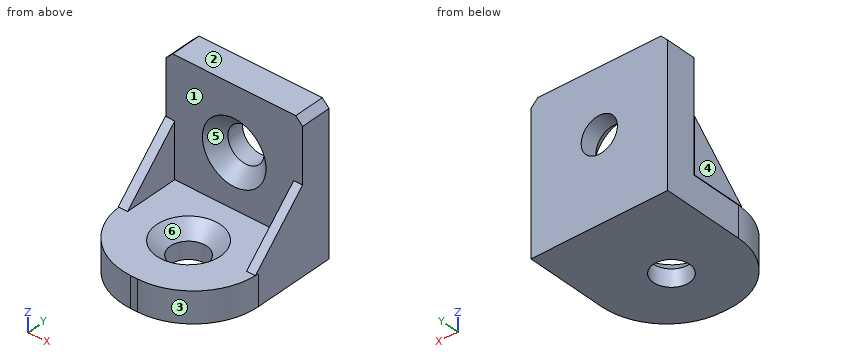
```python
from build123d import *

# Parameters (mm, degrees)
SKETCH_W        = 20
SKETCH_H        = 21.5
PAD_DEPTH       = 21.5
FILLET_R        = 9.5
BOX_W           = 22
BOX_H           = 22
BOX_DEPTH       = 22
SKETCH001_R     = 2.65
POCKET_DEPTH    = 4.5
SKETCH002_R     = 2.65
POCKET001_DEPTH = 4.5
CHAMFER_SIZE    = 2
CHAMFER001_SIZE = 1
SKETCH003_W     = 1.3
SKETCH003_H     = 8
SKETCH003_W_2   = 1.36674
PAD001_DEPTH    = 8
POCKET002_DEPTH = 20.06774


with BuildPart() as part:
    # Sketch → Pad (new body)
    with BuildSketch(Plane.XZ):
        with Locations((0, 10.75)):
            Rectangle(SKETCH_W, SKETCH_H)
    extrude(amount=PAD_DEPTH)

    # Fillet
    fillet_edges = [part.edges().sort_by_distance(p)[0] for p in [
        (10, -21.5, 10.75),
        (-10, -21.5, 10.75),
    ]]
    fillet(fillet_edges, radius=FILLET_R)

    # Box → Box (cut)
    with BuildSketch(Plane(origin=(-11, -4.5, 4.5), x_dir=(1, 0, 0), z_dir=(0, -1, 0))):
        with Locations((11, 11)):
            Rectangle(BOX_W, BOX_H)
    extrude(amount=BOX_DEPTH, mode=Mode.SUBTRACT)

    # Sketch001 (on Face6 of Box) → Pocket (cut)
    with BuildSketch(Plane(origin=(0, -4.5, 12.25), x_dir=(1, 0, 0), z_dir=(0, -1, 0))):
        Circle(SKETCH001_R)
    extrude(amount=-POCKET_DEPTH, mode=Mode.SUBTRACT)

    # Sketch002 (on Face5 of Pocket) → Pocket001 (cut)
    with BuildSketch(Plane(origin=(0, -12.25, 4.5), x_dir=(-1, 0, 0), z_dir=(0, 0, 1))):
        Circle(SKETCH002_R)
    extrude(amount=-POCKET001_DEPTH, mode=Mode.SUBTRACT)

    # Chamfer
    chamfer_edges = [part.edges().sort_by_distance(p)[0] for p in [
        (-2.65, -4.5, 12.25),
        (2.65, -12.25, 4.5),
    ]]
    chamfer(chamfer_edges, length=CHAMFER_SIZE)

    # Chamfer001
    chamfer001_edges = [part.edges().sort_by_distance(p)[0] for p in [
        (10, -2.25, 21.5),
        (-10, -2.25, 21.5),
    ]]
    chamfer(chamfer001_edges, length=CHAMFER001_SIZE)

    # Sketch003 (on Face1 of Chamfer001) → Pad001 (join)
    with BuildSketch(Plane(origin=(0, -4.5, 4.5), x_dir=(1, 0, 0), z_dir=(0, -1, 0))):
        with Locations((9.35, 4)):
            Rectangle(SKETCH003_W, SKETCH003_H)
        with Locations((-9.38337, 4)):
            Rectangle(SKETCH003_W_2, SKETCH003_H)
    extrude(amount=PAD001_DEPTH)

    # Sketch004 (on Face26 of Pad001) → Pocket002 (cut, through all)
    with BuildSketch(Plane(origin=(10, -4.5, 4.5), x_dir=(0, 0, 1), z_dir=(1, 0, 0))):
        Polygon((0, 8), (8, 0), (8, 8), align=None)
    extrude(amount=-POCKET002_DEPTH, mode=Mode.SUBTRACT)


solid = part.part
```
Model file for the job. Use its own axes, mm. Face numbers are marked on the shaded views. A direction names the side the tool comes from. Coordinates: 2 decimals unless noted, no trailing zeros. Order: outer loops, then holes, each group sorted by start corner. A loop starts at its lowest first (then second) coordinate and runs counter-clockwise, first axis right, second up. Notation, with made-up numbers: (24.25, 72.25) - (65.25, 72.25) arc R35 cw to (65.25, 106.25) - close; hole circle Ø10 at (12.25, 9). An arc over 180 degrees is marked (long way). Return JSON: item names as keys, results as strings. Group by question number.
1) Mould opens along X. For the marked faces 3, 4, 5 and 6 say: released by +X, released by -X, zero draft, split by the parting line, or undercut.
2) Saw through at D-D, the plane y = -3.5. Write the cut outline in (x, z), plus the area to 3 significant figures.
3) Saw through at C-C, the plane y = -6.5. Write the cut outline in (x, z).
4) Flat gauge pins, fed straight in: P1, Ø1.5, axis at x = 1.5, y = -6, coming from the +Z side; P2, Ø6, axis at x = 2, z = 8, coming from the -Y side; P3, Ø4, axis at x = 0, y = -12.25, coming from the -Z side; P4, Ø1.5, axis at y = -18, z = 4, coming from the -X side. Where does each tip first touch, or does it go through?
5) Saw through at A-A, the plane x = 0. Write the cut outline in (y, z), plus the area to 3 significant figures.
6) Saw through at B-B, the plane z = 2. Write the cut outline in (x, y), plus the area to 3 significant figures.
7) Tool access for the marked faces 1 and 2: list every direction of +Z, -Z, +X, -X, +Y, -Y with a clear straight run to the whole face (end or side of a thin tool).
8) Probe line 1 (Z direction, x = 0, y = -1.25); line 2 (Y direction, x = 0, z = 1.25); line 3 (X direction, y = -12.25, z = 1.55). List the from-to ranges inside material, lowest first. Write a range as from..to.
Values found:
{
 "1": {"face 3": "released by +X", "face 4": "released by -X", "face 5": "undercut", "face 6": "undercut"},
 "2": {"outline": "(-10, 0) - (10, 0) - (10, 20.5) - (9, 21.5) - (-9, 21.5) - (-10, 20.5) - close; hole circle Ø7.3 at (0, 12.25)", "area": "387 mm²"},
 "3": {"outline": "(-10.07, 4.5) - (-10, 4.5) - (-10, 0) - (10, 0) - (10, 10.5) - (8.7, 10.5) - (8.7, 4.5) - (-8.7, 4.5) - (-8.7, 10.5) - (-10.07, 10.5) - close"},
 "4": {"P1": "stops at z = 4.5", "P2": "stops at y = -4.5", "P3": "passes through", "P4": "stops at x = -8.42"},
 "5": {"outline": "(-21.5, 0) - (-14.9, 0) - (-14.9, 2.5) - (-16.9, 4.5) - (-21.5, 4.5) - close; (-9.6, 0) - (0, 0) - (0, 9.6) - (-2.5, 9.6) - (-4.5, 7.6) - (-4.5, 4.5) - (-7.6, 4.5) - (-9.6, 2.5) - close; (-4.5, 16.9) - (-2.5, 14.9) - (0, 14.9) - (0, 21.5) - (-4.5, 21.5) - close", "area": "118 mm²"},
 "6": {"outline": "(-10, -12) arc R9.5 ccw to (-0.5, -21.5) - (0.5, -21.5) arc R9.5 ccw to (10, -12) - (10, 0) - (-10, 0) - close; hole circle Ø5.3 at (0, -12.25)", "area": "369 mm²"},
 "7": {"face 1": "+Z, -Y", "face 2": "+Z, +X, -X, +Y, -Y"},
 "8": {"line 1": "z = 0..9.6, 14.9..21.5", "line 2": "y = -21.5..-14.9, -9.6..0", "line 3": "x = -10..-2.65, 2.65..10"}
}
